Answer from the drawing. Dimensions are ordinates in mm from the lowest x, y and z of the part. Give positions to 0.01 mm unless a question says otherwise; leave off trailing zeros. Order: outer loops, then holes, each group sorted by start corner. A loop starts at its lowest first (then second) coordinate and runs counter-clockwise, first axis right, second up. Notation, with made-up numbers: M -24.5,14 L 32.5,14 A21 ccw 32.5,50 Z; hole C -36,58.25 d8. An arc over 180 degrees is marked long. One line per item, written item: value.
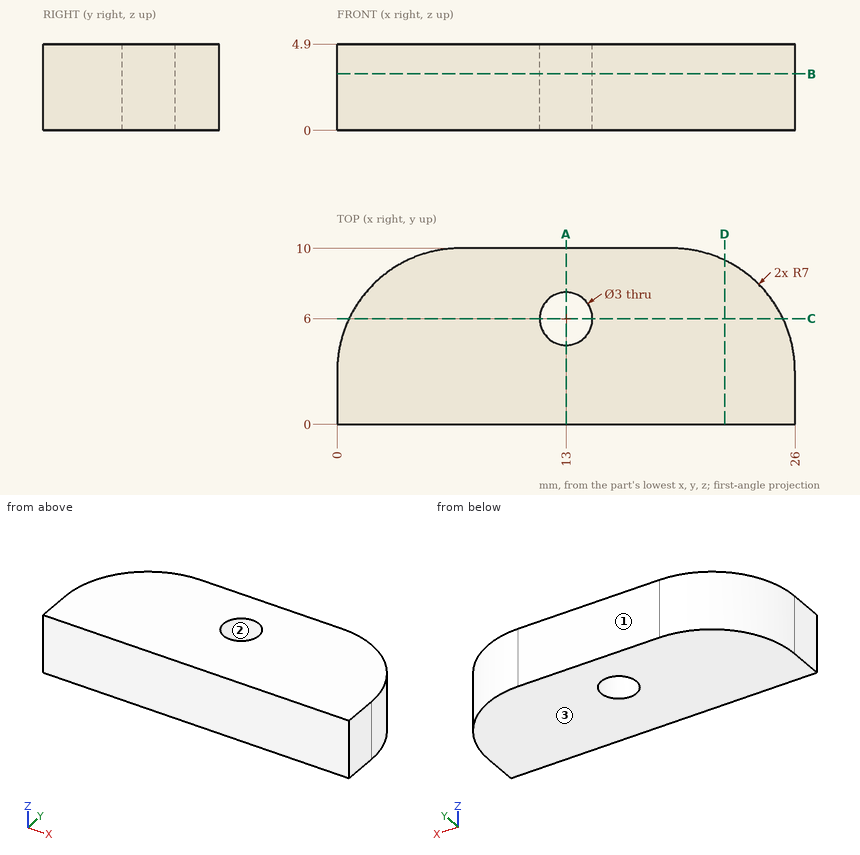
(1) Section A-A, the plane x = 13 is taken. Give the vertices of the cut face in (y, z), then the cut area to 3 significant figures.
Findings:
outline: M 0,0 L 4.5,0 L 4.5,4.9 L 0,4.9 Z; M 7.5,0 L 10,0 L 10,4.9 L 7.5,4.9 Z
area: 34.3 mm^2
(2) Find the intervals of material crossed by probe 1 along Y at (x, z) = (13, 3.85); probe 2 along X at (y, z) = (6, 2.75); probe 3 along Y at (x, z) = (14.25, 2.2), in increasing order. Write a range as from..to.
Findings:
probe 1: y = 0..4.5, 7.5..10
probe 2: x = 0.68..11.5, 14.5..25.32
probe 3: y = 0..5.17, 6.83..10
(3) Given P1, Ø1, axis at x = 3.5, z = 2.5, coming from the +Y side, flat-ended and moving along its own axis, determine where the tip first touches the part or whether it passes through.
Findings:
P1: stops at y = 9.32
(4) Section C-C, the plane y = 6 is taken. Give the vertices of the cut face in (x, z), then the cut area to 3 significant figures.
Findings:
outline: M 0.68,0 L 11.5,0 L 11.5,4.9 L 0.68,4.9 Z; M 14.5,0 L 25.32,0 L 25.32,4.9 L 14.5,4.9 Z
area: 106 mm^2
(5) Section D-D, the plane x = 22 is taken. Give the vertices of the cut face in (y, z), then the cut area to 3 significant figures.
Findings:
outline: M 0,0 L 9.32,0 L 9.32,4.9 L 0,4.9 Z
area: 45.7 mm^2
(6) Determine the mould class of the marked faces 1, 2 and 3 for opening direction Y: pulls with the +Y half, pulls with the -Y half, needs draft (parallel to the pull), parting line crosses it, or undercut.
Findings:
face 1: pulls with the +Y half
face 2: undercut
face 3: needs draft
(7) Section B-B, the plane z = 3.2 is taken. Give the vertices of the cut face in (x, y).
Findings:
outline: M 0,0 L 26,0 L 26,3 A7 ccw 19,10 L 7,10 A7 ccw 0,3 Z; hole C 13,6 d3
